Geometry check sheet. Reference: the model listing, model coordinates, mm. Face numbers are marked on the shaded views. Coordinates: 2 decimals unless noted, no trailing zeros. Write each loop counter-clockwise with the first axis right and the second up, starting at its lowest first coordinate (ties: lowest second). Pieces come first, ordered by that corner, then holes. Notation, with made-up numbers: (23.25, -22) - (45.25, -22) arc R17 ccw to (45.25, -18) - close; hole circle Ø4 at (1.5, 60). An arc over 180 degrees is marked (long way). Answer as a JSON object with one key per item and string values. Group by question number.
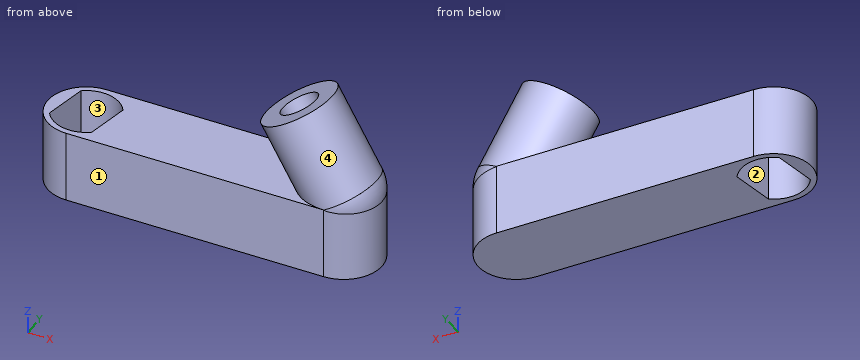
from build123d import *

# Parameters (mm, degrees)
SKETCH011_R     = 8
PAD003_DEPTH    = 18.5
PAD004_DEPTH    = 15
POCKET004_DEPTH = 15.001
SKETCH015_R     = 4
POCKET005_DEPTH = 20


with BuildPart() as part:
    # Sketch011 (on DatumPlane) → Pad003 (new body)
    with BuildSketch(Plane(origin=(44.455971, 0, 0), x_dir=(0.866025, 0, 0.5), z_dir=(-0.5, 0, 0.866025))):
        Circle(SKETCH011_R)
    extrude(amount=-PAD003_DEPTH)

    # Sketch012 → Revolution001 (revolve)
    with BuildSketch(Plane.XZ):
        with BuildLine():
            ThreePointArc((46.777767, -20.02147), (51.635418, -23.748877), (57.705971, -22.949673))
            Line((53.705971, -16.02147), (57.705971, -22.949673))
            Line((46.777767, -20.02147), (53.705971, -16.02147))
        make_face()
    revolve(axis=Axis((44.455971, 0, 0), (-0.5, 0, 0.866025)))

    # Sketch013 (on DatumPlane) → Pad004 (join)
    with BuildSketch(Plane.XY.offset(-16)):
        with BuildLine():
            ThreePointArc((0, 8), (-8, 0), (0, -8))
            Line((0, -8), (53.693575, -8))
            ThreePointArc((53.693575, -8), (61.693575, 0), (53.693575, 8))
            Line((0, 8), (53.693575, 8))
        make_face()
    extrude(amount=-PAD004_DEPTH)

    # Sketch014 (on DatumPlane) → Pocket004 (cut, through all)
    with BuildSketch(Plane.XY.offset(-16)):
        with BuildLine():
            ThreePointArc((5.804447, 3.551769), (1.32757, 6.674146), (-4.003406, 5.502672))
            Line((-5.804447, -3.551769), (-4.003406, 5.502672))
            ThreePointArc((-5.804447, -3.551769), (-1.32757, -6.674146), (4.003406, -5.502672))
            Line((4.003406, -5.502672), (5.804447, 3.551769))
        make_face()
    extrude(amount=-POCKET004_DEPTH, mode=Mode.SUBTRACT)

    # Sketch015 (on Face6 of Pocket004) → Pocket005 (cut)
    with BuildSketch(Plane(origin=(44.455971, 0, 0), x_dir=(0.866025, 0, 0.5), z_dir=(-0.5, 0, 0.866025))):
        Circle(SKETCH015_R)
    extrude(amount=-POCKET005_DEPTH, mode=Mode.SUBTRACT)


with BuildPart() as part_1:
    # Body002 placement: moved
    add(part.part.moved(Location((0, 0, 31))))


solid = part_1.part
(1) Draft check along Y on the marked faces 1, 2, 3 and 4. Enter one of: +Y half, -Y half, draft (parallel to the pull), parting line (faces both ways), or undercut.
(2) Gauge pin test, flat ends, axial feed: pin 1 (5 mm diameter, centred on x = 12, y = -3.5, fed in from +Z); pin 2 (1 mm diameter, centred on y = -3, z = 14, fed in from -X); pin 3 (3 mm diameter, centred on x = 52.5, y = -5.5, fed in from +Z). Record the tip position at first contact, or that the pin passes through.
(3) Section check A-A (z = 10). Record the cut outline in (x, y), and give its area (3 significant figures).
(4) Material ranges on L1, parallel to X at y = 1.5, z = 12; L2, parallel to X at y = -1.5, z = 2.5; L3, parallel to Y at x = 52, z = 25 (3 decimals), recorded low to high. Write a range as [from, to].
(5) Section check B-B (x = 15). Record the cut outline in (y, z), and give its area (3 significant figures).
Conclusion:
{
 "1": {"face 1": "-Y half", "face 2": "undercut", "face 3": "undercut", "face 4": "parting line"},
 "2": {"pin 1": "stops at z = 15", "pin 2": "stops at x = -7.6", "pin 3": "stops at z = 32.24"},
 "3": {"outline": "(0, -8) - (53.69, -8) arc R8 ccw to (53.69, 8) - (0, 8) arc R8 ccw to start; hole (-5.8, -3.55) arc R6.8 ccw to (4, -5.5) - (5.8, 3.55) arc R6.8 ccw to (-4, 5.5) - close", "area": "938 mm^2"},
 "4": {"L1": "x = [-7.86, -4.8], [5.4, 51.14], [51.55, 61.55]", "L2": "x = [-7.86, -5.4], [4.8, 61.55]", "L3": "y = [-7.177, -1.875], [1.875, 7.177]"},
 "5": {"outline": "(-8, 0) - (8, 0) - (8, 15) - (-8, 15) - close", "area": "240 mm^2"}
}
